```python
from build123d import *

# Parameters (mm, degrees)
F0_W     = 35.56
F0_H     = 17.78
F1_DEPTH = 0.635
F2_R     = 0.635
F3_DEPTH = 20.32


with BuildPart() as f1:
    # F0 (on Top) → F1 (new body)
    with BuildSketch(Plane.XY):
        with Locations((-17.78, -8.89)):
            Rectangle(F0_W, F0_H)
    extrude(amount=-F1_DEPTH)

    # F2 (on Top) → F3 (join)
    with BuildSketch(Plane.XY):
        with Locations((-34.29, -1.27)):
            Circle(F2_R)
        with Locations((-34.29, -16.51)):
            Circle(F2_R)
        with Locations((-1.27, -16.51)):
            Circle(F2_R)
        with Locations((-1.27, -1.27)):
            Circle(F2_R)
    extrude(amount=-F3_DEPTH)


solid = f1.part
```
CAD build for the part. Positions are in the model's coordinates, mm. A direction names the side the tool comes from. Round coordinates to 2 decimals unless told otherwise and drop trailing zeros. Loops run counter-clockwise (first coordinate to the right, second up) from the corner with the lowest first, then second, coordinate; pieces in that order, holes last. Notation, with made-up numbers: M -38.75,-34.5 L -21.75,-34.5 A38 ccw -21.75,3.5 Z; hole C -10.75,0.5 d10. An arc over 180 degrees is marked long. Use a Markdown table: item, result. Add a question column.
(1) Cut at D-D (x = -6). Give the cut face in (y, z) (3 decimals).
(2) Flat gauge pins, fed straight in: pin 1 (1 mm diameter, centred on x = -21, y = -15.5, fed in from +Z); pin 2 (2 mm diameter, centred on x = -13.5, y = -4, fed in from -Z) (3 decimals). Where does each tip first touch, or does it go through?
(3) Which spindle directions (+Z, -Z, +X, -X, +Y, -Y) get a long thin tool onto all of the face, cutting with end or side? Do faces 3 (the face through (-1.3, -16.5, -20.32)), 4 (the face through (-1.41, -17.13, -10.34)). Say none if no direction does.
(4) Cut at A-A (y = -16.51). Give the cut face in (x, z) (3 decimals).
(5) Cut at B-B (x = -34.29). Give the cut face in (y, z) (3 decimals), and give its area (3 significant figures).
(6) Drill centre lines: line 1 (Z direction, x = -12.5, y = -8.25) (3 decimals); line 2 (X direction, y = -1, z = -4.75); line 3 (X direction, y = -1.5, z = -18.25). Where is each one in solid material? Low to high.
(7) Cut at C-C (z = -1.5). Give the cut face in (x, y) (3 decimals), and give its area (3 significant figures).
(8) Pull direction X, two halves, no side cores. Call faces 1 (the face through (-1, -1, -20.32)), 2 (the face through (-33.684, -1.079, -10.34)): +X half, -X half, draft (parallel to the pull), parting line (faces both ways), or undercut.
Geometry says:
| question | item | result |
|---|---|---|
| 1 | outline | M -17.78,-0.635 L 0,-0.635 L 0,0 L -17.78,0 Z |
| 2 | pin 1 | stops at z = 0 |
| 2 | pin 2 | stops at z = -0.635 |
| 3 | face 3 | -Z, +X, -X, +Y, -Y |
| 3 | face 4 | -Z |
| 4 | outline | M -35.56,-0.635 L -34.925,-0.635 L -34.925,-20.32 L -33.655,-20.32 L -33.655,-0.635 L -1.905,-0.635 L -1.905,-20.32 L -0.635,-20.32 L -0.635,-0.635 L 0,-0.635 L 0,0 L -35.56,0 Z |
| 5 | outline | M -17.78,-0.635 L -17.145,-0.635 L -17.145,-20.32 L -15.875,-20.32 L -15.875,-0.635 L -1.905,-0.635 L -1.905,-20.32 L -0.635,-20.32 L -0.635,-0.635 L 0,-0.635 L 0,0 L -17.78,0 Z |
| 5 | area | 61.3 mm² |
| 6 | line 1 | z = -0.635 to 0 |
| 6 | line 2 | x = -34.86 to -33.72, -1.84 to -0.7 |
| 6 | line 3 | x = -34.88 to -33.7, -1.86 to -0.68 |
| 7 | outline | C -34.29,-16.51 d1.27; C -34.29,-1.27 d1.27; C -1.27,-16.51 d1.27; C -1.27,-1.27 d1.27 |
| 7 | area | 5.07 mm² |
| 8 | face 1 | draft |
| 8 | face 2 | undercut |
